Input: part model. Units: mm. Frame: model coordinates. A direction names the side the tool comes from. Round coordinates to 2 decimals unless told otherwise and drop trailing zeros. Loops run counter-clockwise (first coordinate to the right, second up) from the corner with the lowest first, then second, coordinate; pieces in that order, holes last. Notation, with made-up numbers: (72, 49.25) -> (119, 49.25) arc R22 ccw to (119, 69.25) -> close; hole circle Ø3 at (-24, -30). An arc over 180 degrees is marked (long way). Answer in a Markdown table with one row per item. Add a question column.
Q1. Section B-B, the plane z = -5.5. Output: boundary loops of the cut face in (x, y).
Q2. Reachability of faces 1 (the face through (10, -10, 0)), 2 (the face through (-10, -9, 0)), 3 (the face through (0, -6, 17)), 4 (the face through (-1.08, 4.88, -10.21)) from +Z, -Z, +X, -X, +Y, -Y: full face, straight path, thin tool, end or side. Return the list, or none.
Q3. Pin query (flat end, axial travel): pin 1 (3.5 mm diameter, centred on x = -6.5, y = 5.5, fed in from -Z); pin 2 (5 mm diameter, centred on x = 7, y = -9, fed in from +Z); pin 3 (3 mm diameter, centred on x = -6, z = -16, fed in from +Y); pin 4 (3.5 mm diameter, centred on x = -6, y = -7.5, fed in from -Z). Return the tip coordinate at first contact, or that it passes through.
Q4. Section A-A, the plane z = 15.5. Output: boundary loops of the cut face in (x, y).
Q5. Ray query, L1, parallel to X at y = 8.2, z = 24; L2, parallel to Z at x = 0, y = -7.55. Return the intervals inside material, ascending. Write a range as from..to.
Q6. Mould query, pull axis X, two halves, no side actions, for faces 5 (the face through (-10, 9, 0)), 6 (the face through (-1.18, -5.31, -6.56)), 7 (the face through (-1.301, 9.042, 29.857)). Classes: pulls with the +X half, pulls with the -X half, needs draft (parallel to the pull), parting line crosses it, or undercut.
Q7. Section C-C, the plane z = -15. Output: boundary loops of the cut face in (x, y), and give its area (3 significant figures).
Solid Edge part; units mm, degrees
sketch "Sketch1" plane through (0, 0, 0) normal (0, -1, 0) x (1, 0, 0)
  line L0 (-12, 0) -> (12, 0)
  line L1 (12, 0) -> (12, 24)
  line L2 (-12, 0) -> (-12, 24)
  arc A0 (12, 24) -> (-12, 24) centre (0, 24) ccw
  circle A1 centre (0, 24) radius 6
  dimension "D1" = 12
extrude "Protrusion1" add sketch "Sketch1" along normal mid plane 24
sketch "Sketch2" plane through (12, 0, 12) normal (1, 0, 0) x (0, 1, 0)
  line L0 (-6, 24) -> (6, 24)
  line L1 (6, 24) -> (6, -2)
  line L2 (6, -2) -> (-6, -2)
  line L3 (-6, -2) -> (-6, 24)
  dimension "D1" = 6
extrude "ExtrudedCutout_1" cut sketch "Sketch2" along normal mid plane 367.3731
sketch "Sketch3" plane through (0, 0, 0) normal (0, -1, 0) x (1, 0, 0)
  line L0 (12, 0) -> (0, 0)
  line L1 (5, -13.3397) -> (0, -22)
  line L2 (5, -7) -> (5, -13.3397)
  line L3 (12, 0) -> (5, -7)
  dimension "D1" = 5
revolve "RevolvedProtrusion1" add sketch "Sketch3" angle 360 about axis through (0, 0, 0) along (0, 0, -1)
properties part number "12" material "Fe 410 W"
Answer block:
| question | item | result |
|---|---|---|
| 1 | outline | circle Ø13 at (0, 0) |
| 2 | face 1 | -Z, +X, -Y |
| 2 | face 2 | -Z, -X, -Y |
| 2 | face 3 | +Z, +X, -X |
| 2 | face 4 | -Z |
| 3 | pin 1 | z = -5.24 |
| 3 | pin 2 | z = 35.12 |
| 3 | pin 3 | through |
| 3 | pin 4 | z = -4.15 |
| 4 | outline | (-12, -12) -> (12, -12) -> (12, -6) -> (-12, -6) -> close; (-12, 6) -> (12, 6) -> (12, 12) -> (-12, 12) -> close |
| 5 | L1 | -12..-6, 6..12 |
| 5 | L2 | -4.45..18, 30..36 |
| 6 | face 5 | needs draft |
| 6 | face 6 | parting line crosses it |
| 6 | face 7 | undercut |
| 7 | outline | circle Ø8.08 at (0, 0) |
| 7 | area | 51.3 mm^2 |
